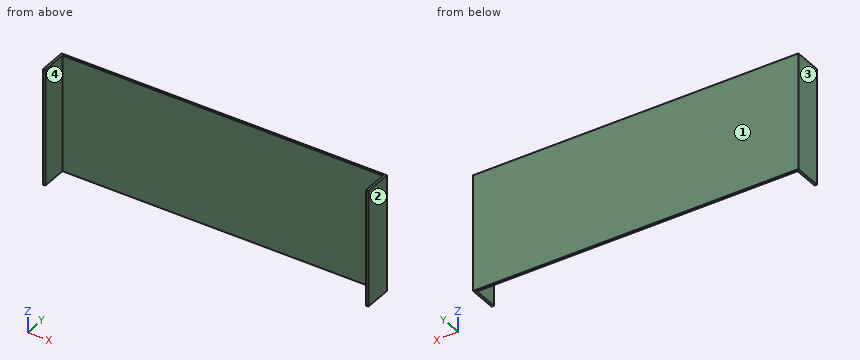
from build123d import *

# Parameters (mm, degrees)
SKETCH1_W           = 700
SKETCH1_H           = 250
BOSS_EXTRUDE1_DEPTH = 60
SHELL1_T            = -5
SKETCH3_W           = 690
SKETCH3_H           = 55
CUT_EXTRUDE1_DEPTH  = 435.281015012


with BuildPart() as part:
    # Sketch1 → Boss-Extrude1 (new body)
    with BuildSketch(Plane(origin=(0, 0, 0), x_dir=(1, 0, 0), z_dir=(0, 1, 0))):
        Rectangle(SKETCH1_W, SKETCH1_H)
    extrude(amount=BOSS_EXTRUDE1_DEPTH)

    # Shell1
    shell1_openings = [part.faces().sort_by_distance(p)[0] for p in [
        (0, 0, 0),
    ]]
    offset(amount=SHELL1_T, openings=shell1_openings, kind=Kind.INTERSECTION)

    # Sketch3 → Cut-Extrude1 (cut, through all)
    with BuildSketch(Plane.XY.offset(125)):
        with Locations((0, 27.5)):
            Rectangle(SKETCH3_W, SKETCH3_H)
    extrude(amount=-CUT_EXTRUDE1_DEPTH, mode=Mode.SUBTRACT)


solid = part.part
Geometry check sheet. Reference: the model listing, model coordinates, mm. Face numbers are marked on the shaded views. Coordinates: 2 decimals unless noted, no trailing zeros. Write each loop counter-clockwise with the first axis right and the second up, starting at its lowest first coordinate (ties: lowest second). Pieces come first, ordered by that corner, then holes. Notation, with made-up numbers: (71.25, -5.75) -> (80.25, -5.75) arc R20 ccw to (80.25, 24.25) -> close; hole circle Ø6 at (-25, 82.5). An arc over 180 degrees is marked (long way). One line per question, with ' | ' between items.
1. Cross-section at C-C on x = -77.5. Record the cut outline in (y, z).
Answers:
outline: (55, -125) -> (60, -125) -> (60, 125) -> (55, 125) -> close
2. Cross-section at B-B on z = -105.5. Record the cut outline in (x, y), and give its area (3 significant figures).
Answers:
outline: (-350, 0) -> (-345, 0) -> (-345, 55) -> (345, 55) -> (345, 0) -> (350, 0) -> (350, 60) -> (-350, 60) -> close | area: 4,050 mm²
3. Depth check by flat-ended pin: pin 1 Ø8 at (x, z) = (-211.5, -14) entering from -Y. Enter the tip coordinate at first touch or a pass-through.
Answers:
pin 1: stops at y = 55
4. Cross-section at A-A on y = 25.5. Record the cut outline in (x, z), and give its area (3 significant figures).
Answers:
outline: (-350, -125) -> (-345, -125) -> (-345, 125) -> (-350, 125) -> close; (345, -125) -> (350, -125) -> (350, 125) -> (345, 125) -> close | area: 2,500 mm²
5. Draft check along X on the marked faces 1, 2, 3 and 4. Enter one of: +X half, -X half, draft (parallel to the pull), parting line (faces both ways), or undercut.
Answers:
face 1: draft | face 2: +X half | face 3: -X half | face 4: undercut
6. Thickness scan on probe 1 along X at (y, z) = (52, 106.5); probe 2 along Y at (x, z) = (-43, 13.5). Record the ranges inside material, lowest first. Write a range as from..to.
Answers:
probe 1: x = -350..-345, 345..350 | probe 2: y = 55..60
